from build123d import *

# Parameters (mm, degrees)
SALIENTE_EXTRUIR1_DEPTH = 400


with BuildPart() as part:
    # Croquis1 → Saliente-Extruir1 (new body)
    with BuildSketch(Plane(origin=(0, 0, 0), x_dir=(0, 0, -1), z_dir=(1, 0, 0))):
        with BuildLine():
            Line((-3, 0), (-255, 0))
            Line((-255, 0), (-255, -3))
            Line((-255, -3), (-3, -3))
            Line((-3, -3), (-3, -157))
            ThreePointArc((-3, -157), (-1.242640687, -161.242640687), (3, -163))
            Line((3, -163), (168.8, -163))
            Line((168.8, -163), (168.8, -160))
            Line((168.8, -160), (3, -160))
            ThreePointArc((3, -160), (0.878679656, -159.121320344), (0, -157))
            Line((0, -157), (0, -3))
            ThreePointArc((0, -3), (-0.878679656, -0.878679656), (-3, 0))
        make_face()
    extrude(amount=SALIENTE_EXTRUIR1_DEPTH)


solid = part.part
The listing builds one solid part. Answer for the finished solid, in the listing's coordinates (mm). A direction names the side the tool comes from. Give positions to 0.01 mm unless a question says otherwise; leave off trailing zeros. Order: outer loops, then holes, each group sorted by start corner. A loop starts at its lowest first (then second) coordinate and runs counter-clockwise, first axis right, second up. Notation, with made-up numbers: (0, 72) - (31, 72) arc R24 ccw to (31, 93) - close; hole circle Ø4 at (20, -15). An arc over 180 degrees is marked (long way). One line per item, written item: value. Start each with the question number.
1) A cutting plane is placed at C-C on z = 101. Give the vertices of the cut face in (x, y).
2) A cutting plane is placed at B-B on y = -21.5. Give the vertices of the cut face in (x, z), then the cut area to 3 significant figures.
3) A tool of negligible diameter and unlimited length cuts with its end or side. For faces 1 (the face through (197, -163, -85)), 2 (the face through (197, -160, -87)), 3 (the face through (197, -79, 3)), from which of +Z, -Z, +X, -X, +Y, -Y can it reach the whole face along a straight path? Write none if from no direction.
4) Given pin 1 Ø12 at (x, y) = (211.5, -118) entering from -Z; pin 2 Ø10 at (x, y) = (307, -110) entering from +Z, each flat-ended and moving along its own axis, determine where each tip first touches the part or whether it passes through.
5) Find the intervals of material crossed by L1, parallel to Y at x = 88, z = -5; L2, parallel to Y at x = 141, z = 235.5; L3, parallel to Z at x = 247, y = -153.5, in increasing order.
6) A cutting plane is placed at A-A on x = 81. Give the vertices of the cut face in (y, z), then the cut area to 3 significant figures.
Answer sheet:
1. outline: (0, -3) - (400, -3) - (400, 0) - (0, 0) - close
2. outline: (0, 0) - (400, 0) - (400, 3) - (0, 3) - close
2. area: 1,200 mm2
3. face 1: +Z, -Z, +X, -X, -Y
3. face 2: -Z, +X, -X, +Y
3. face 3: +Z, +X, -X, -Y
4. pin 1: stops at z = 0
4. pin 2: stops at z = 3
5. L1: y = -163 to -160
5. L2: y = -3 to 0
5. L3: z = 0 to 3
6. outline: (-163, -168.8) - (-160, -168.8) - (-160, -3) arc R3 cw to (-157, 0) - (-3, 0) arc R3 ccw to (0, 3) - (0, 255) - (-3, 255) - (-3, 3) - (-157, 3) arc R6 ccw to (-163, -3) - close
6. area: 1,740 mm2
